Could you check a few things on this model? Use its own coordinates, in mm. Give positions to 0.01 mm unless a question says otherwise; leave off trailing zeros. Order: outer loops, then holes, each group sorted by start corner. A loop starts at its lowest first (then second) coordinate and runs counter-clockwise, first axis right, second up. Notation, with made-up numbers: (86, 82.5) - (92, 82.5) arc R25 cw to (92, 98.5) - close; hole circle Ø11 at (-9, 89.25). An arc over 180 degrees is marked (long way). One line per question, with ' | ' between items. Start each with the question number.
1. Imagine slicing it at D-D (y = -3.8). Please give me the cut outline in (x, z), and give its area (3 significant figures).
2. Imagine slicing it at B-B (x = 55). Please give me the cut outline in (y, z).
3. Imagine slicing it at A-A (z = 10). Give the number of separate pieces and of enclosed holes in the cut face, and give its area (3 significant figures).
4. I need wall thicknesses on probe 1 along Z at (x, y) = (35, -1.1); probe 2 along Z at (x, y) = (47.5, -1.25); probe 3 along Z at (x, y) = (56, -3.1). Which ranges of each line are inside material? Lowest first, please. Write a range as from..to.
5. Imagine slicing it at C-C (z = 74). Please give me the cut outline in (x, y).
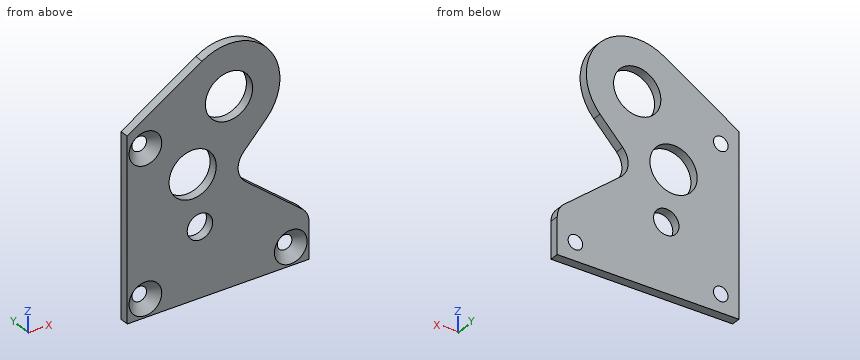
```python
from build123d import *

# Parameters (mm, degrees)
F0_R     = 4
F0_R_2   = 7
F0_R_3   = 13
F1_DEPTH = 5
F2_SIZE  = 4.99999
F3_R     = 10


# Not quite as in the source:
# - a fillet or chamfer is up to 0.001 mm smaller than in the source, because OpenCascade refuses the exact size


with BuildPart() as f1:
    # F0 (on Front) → F1 (new body)
    with BuildSketch(Plane.XZ):
        with BuildLine():
            Line((0, 100), (0, 0))
            Line((0, 0), (100, 0))
            Line((100, 0), (100, 25))
            Line((100, 25), (65.0521931045, 53.4719299169))
            ThreePointArc((65.0521931045, 53.4719299169), (61.0252955601, 61.2544381602), (63.9626496251, 69.51005985))
            Line((63.9626496251, 69.51005985), (76.4587100452, 82.8834840181))
            ThreePointArc((76.4587100452, 82.8834840181), (77.6106511533, 119.803925318), (41.1521770426, 125.7390428077))
            Line((41.1521770426, 125.7390428077), (0, 100))
        make_face()
        with Locations((10, 10)):
            Circle(F0_R, mode=Mode.SUBTRACT)
        with Locations((40, 38)):
            Circle(F0_R_2, mode=Mode.SUBTRACT)
        with Locations((90, 10)):
            Circle(F0_R, mode=Mode.SUBTRACT)
        with Locations((10, 90)):
            Circle(F0_R, mode=Mode.SUBTRACT)
        with Locations((36, 67.24)):
            Circle(F0_R_3, mode=Mode.SUBTRACT)
        with Locations((56, 102)):
            Circle(F0_R_3, mode=Mode.SUBTRACT)
    extrude(amount=F1_DEPTH)

    # F2 (size 5 in the source; OpenCascade refuses exactly that, so slightly less here)
    f2_edges = [f1.edges().sort_by_distance(p)[0] for p in [
        (6, -5, 10),
        (86, -5, 10),
        (6, -5, 90),
    ]]
    chamfer(f2_edges, length=F2_SIZE)

    # F3
    f3_edges = [f1.edges().sort_by_distance(p)[0] for p in [
        (100, -2.5, 25),
    ]]
    fillet(f3_edges, radius=F3_R)


solid = f1.part
```
Results found:
1) outline: (0, 0) - (100, 0) - (100, 20.25) arc R10 ccw to (96.32, 28) - (65.05, 53.47) arc R11 cw to (63.96, 69.51) - (76.46, 82.88) arc R28 ccw to (41.15, 125.74) - (0, 100) - close; hole circle Ø15.6 at (10, 10); hole circle Ø15.6 at (10, 90); hole circle Ø26 at (36, 67.24); hole circle Ø14 at (40, 38); hole circle Ø26 at (56, 102); hole circle Ø15.6 at (90, 10) | area: 8,010 mm2
2) outline: (-5, 0) - (0, 0) - (0, 89.04) - (-5, 89.04) - close; (-5, 114.96) - (0, 114.96) - (0, 129.98) - (-5, 129.98) - close
3) separate pieces: 3 | enclosed holes: 0 | area: 370 mm2
4) probe 1: z = 0..33.1, 42.9..54.28, 80.2..121.89 | probe 2: z = 0..61.18, 73.3..92.16, 111.84..128.68 | probe 3: z = 0..89, 115..130
5) outline: (0, -5) - (24.9, -5) - (24.9, 0) - (0, 0) - close; (47.1, -5) - (68.16, -5) - (68.16, 0) - (47.1, 0) - close
